Can you work these out from the model? Positions are in its coordinate system, mm. Give positions to 0.01 mm unless a question says otherwise; leave off trailing zeros. Loops run counter-clockwise (first coordinate to the right, second up) from the corner with the lowest first, then second, coordinate; pieces in that order, holes last. Notation, with made-up numbers: (-14, 25.5) - (23, 25.5) arc R21 cw to (23, 44.5) - close; hole circle Ø10 at (-19.5, 6.5). An arc over 180 degrees is marked (long way). Answer in a Markdown table with one row per item.
from build123d import *

# Parameters (mm, degrees)
M3_GEWINDEBOHRUNG1_D = 2.5
KREISMUSTER2_COUNT   = 4


with BuildPart() as part:
    # Skizze1 → Rotation1 (revolve)
    with BuildSketch(Plane.XY, mode=Mode.PRIVATE) as rotation1_sk:
        Polygon((-31.181837907, 20), (-31.181837907, 14), (-29.181837907, 14), (-15.181837907, 14), (-15.181837907, 20), align=None)
    revolve(rotation1_sk.sketch.rotate(Axis((-37.668433178, 0, 0), (1, 0, 0)), 90), axis=Axis((-37.668433178, 0, 0), (1, 0, 0)))

    # M3 Gewindebohrung1 (through all)
    with Locations(Plane(origin=(-15.181837907, 0, 0), x_dir=(0, 0, -1), z_dir=(1, 0, 0))):
        with Locations((0, 17)):
            m3_gewindebohrung1 = Hole(M3_GEWINDEBOHRUNG1_D / 2)

    # Kreismuster2: M3 Gewindebohrung1 ×4 about axis
    kreismuster2_axis = Axis((0, 0, 0), (1, 0, 0))
    for i in range(1, KREISMUSTER2_COUNT):
        add(m3_gewindebohrung1.rotate(kreismuster2_axis, i * 360 / KREISMUSTER2_COUNT), mode=Mode.SUBTRACT)


solid = part.part
Q1. Imagine slicing it at D-D, the plane y = 5.5. Write out the boundary of the cut face in (x, z).
Checked values:
| item | result |
|---|---|
| outline | (-31.18, -19.23) - (-15.18, -19.23) - (-15.18, -12.87) - (-31.18, -12.87) - close; (-31.18, 12.87) - (-15.18, 12.87) - (-15.18, 19.23) - (-31.18, 19.23) - close |
Q2. If I drill on line 1 (Y direction, x = -25.75, z = 0); line 2 (Y direction, x = -30.5, z = 0.5); line 3 (Z direction, x = -24.75, y = -16), over which ranges is the centre line in solid material (lowest first)? Write a range as [from, to].
Checked values:
| item | result |
|---|---|
| line 1 | y = [-20, -18.25], [-15.75, -14], [14, 15.75], [18.25, 20] |
| line 2 | y = [-19.99, -18.15], [-15.85, -13.99], [13.99, 15.85], [18.15, 19.99] |
| line 3 | z = [-12, -0.75], [0.75, 12] |
Q3. Imagine slicing it at A-A, the plane y = 0. Write out the boundary of the cut face in (x, z).
Checked values:
| item | result |
|---|---|
| outline | (-31.18, -20) - (-15.18, -20) - (-15.18, -18.25) - (-31.18, -18.25) - close; (-31.18, -15.75) - (-15.18, -15.75) - (-15.18, -14) - (-31.18, -14) - close; (-31.18, 14) - (-15.18, 14) - (-15.18, 15.75) - (-31.18, 15.75) - close; (-31.18, 18.25) - (-15.18, 18.25) - (-15.18, 20) - (-31.18, 20) - close |
Q4. Imagine slicing it at B-B, the plane z = 17.5. Write out the boundary of the cut face in (x, y), and give its area (3 significant figures).
Checked values:
| item | result |
|---|---|
| outline | (-31.18, -9.68) - (-15.18, -9.68) - (-15.18, -1.15) - (-31.18, -1.15) - close; (-31.18, 1.15) - (-15.18, 1.15) - (-15.18, 9.68) - (-31.18, 9.68) - close |
| area | 273 mm² |
Q5. If we mould it in two halves opening along Z, with no side actions, what happens to faces 1 (the face through (-23.294, -0.672, 18.054)), 2 (the face through (-23.294, 0.672, -18.054)), 3 (the face through (-15.182, -12, 8)), 4 (the face through (-23.29, -0.88, -19.98))? For each: released by +Z, released by -Z, zero draft, split by the parting line, or undercut.
Checked values:
| item | result |
|---|---|
| face 1 | undercut |
| face 2 | undercut |
| face 3 | zero draft |
| face 4 | split by the parting line |
Q6. Imagine slicing it at C-C, the plane x = -23.25. Write out the boundary of the cut face in (y, z).
Checked values:
| item | result |
|---|---|
| outline | circle Ø40 at (0, 0); hole circle Ø2.5 at (-17, 0); hole circle Ø28 at (0, 0); hole circle Ø2.5 at (0, -17); hole circle Ø2.5 at (0, 17); hole circle Ø2.5 at (17, 0) |
Q7. For pin 1 (5 mm diameter, centred on x = -21.5, z = -8.5, fed in from +Y); pin 2 (3 mm diameter, centred on y = -1, z = 13.5, fed in from -X); pin 3 (4 mm diameter, centred on x = -27.5, y = -2.5, fed in from -Z); pin 4 (5 mm diameter, centred on x = -23.5, y = -7, fed in from -Z), each with a flat end and sliding along its axis, tell me the tip position at first contact or that it passes through.
Checked values:
| item | result |
|---|---|
| pin 1 | stops at y = 19.08 |
| pin 2 | stops at x = -31.18 |
| pin 3 | stops at z = -19.99 |
| pin 4 | stops at z = -19.49 |
